Could you check a few things on this model? Use its own coordinates, in mm. A direction names the side the tool comes from. Coordinates: 2 decimals unless noted, no trailing zeros. Write each loop counter-clockwise with the first axis right and the second up, starting at its lowest first coordinate (ties: lowest second). Pieces come first, ordered by that corner, then holes.
Item 1: For P1, Ø0.9, axis at y = -1.5, z = 137.5, coming from the +X side; P2, Ø0.6, axis at x = -3.5, y = -1.5, coming from the -Z side; P3, Ø4.5, axis at x = -1, z = 137, coming from the +Y side; P4, Ø1.5, axis at y = -2, z = 116, coming from the +X side, each with a flat end and sliding along its axis, tell me the tip position at first contact or that it passes through.
Item 2: Which directions (+Z, -Z, +X, -X, +Y, -Y) give clear straight access to the entire face, cutting with the end or side of a thin tool? Please do faces 4 (the flat face through (-1, 2.54, 137)), 5 (the flat face through (-1, -2.996, 137)), 6 (the flat face through (2.952, -2, 137)).
Item 3: If I drill on probe 1 along Y at (x, z) = (0.5, 44); probe 2 along Y at (x, z) = (0.5, 134); probe 3 along Z at (x, y) = (2.5, 2.25), over which ranges is the centre line in solid material (lowest first)?
Item 4: I want a section at B-B on z = 70. Please give me the cut outline in (x, y).
Item 5: Thinking about a two-plate mould opening in Z: for faces 1 (the flat face through (0, 0, 0)), 2 (the cylindrical face through (4, 1.3, 61.4)), 3 (the cylindrical face through (-0.5, 1.25, 134.75)), which applies, +Z half, -Z half, draft (parallel to the pull), parting line (faces both ways), or undercut?
Item 6: I want a section at A-A on x = -0.5. Please give me the cut outline in (y, z).
from build123d import *

# Parameters (mm, degrees)
F0_R     = 4.20629
F1_DEPTH = 124.6124
F2_W     = 7.158407
F2_H     = 2.996312
F3_DEPTH = 25.4
F4_R     = 2.036724
F5_DEPTH = 2.54


with BuildPart() as f1:
    # F0 (on Top) → F1 (new body)
    with BuildSketch(Plane.XY):
        Circle(F0_R)
    extrude(amount=F1_DEPTH)

    # F2 (on face) → F3 (join)
    with BuildSketch(Plane.XY.offset(124.6124)):
        with Locations((-0.627087, -1.498156)):
            Rectangle(F2_W, F2_H)
    extrude(amount=F3_DEPTH)

    # F4 (on face) → F5 (join)
    with BuildSketch(Plane(origin=(0, 0, 0), x_dir=(-1, 0, 0), z_dir=(0, 1, 0))):
        with Locations((0.938338, 136.737749)):
            Circle(F4_R)
    extrude(amount=F5_DEPTH)


solid = f1.part
Response values:
1. P1: stops at x = 2.95
1. P2: stops at z = 0
1. P3: stops at y = 2.54
1. P4: stops at x = 4.02
2. face 4: +Z, +X, -X, +Y
2. face 5: +Z, +X, -X, -Y
2. face 6: +Z, +X, +Y, -Y
3. probe 1: y = -4.18 to 4.18
3. probe 2: y = -3 to 0
3. probe 3: z = 0 to 124.61
4. outline: circle Ø8.41 at (0, 0)
5. face 1: -Z half
5. face 2: draft
5. face 3: undercut
6. outline: (-4.18, 0) - (4.18, 0) - (4.18, 124.61) - (0, 124.61) - (0, 134.75) - (2.54, 134.75) - (2.54, 138.73) - (0, 138.73) - (0, 150.01) - (-3, 150.01) - (-3, 124.61) - (-4.18, 124.61) - close
